Could you check a few things on this model? Use its own coordinates, in mm. A direction names the side the tool comes from. Coordinates: 2 decimals unless noted, no trailing zeros. Order: outer loops, then holes, each group sorted by start corner. A loop starts at its lowest first (then second) coordinate and runs counter-clockwise, first axis right, second up. Notation, with made-up numbers: (88.5, 31) -> (135.5, 31) arc R29 cw to (135.5, 62) -> close; hole circle Ø7 at (-19, 32). An arc over 180 degrees is marked (long way). Use a Markdown table: item, result. Add a question column.
1) If I drill on L1, parallel to Y at x = 0, z = 1.2; L2, parallel to X at y = 0, z = 6.75 (3 decimals), over which ranges is the centre line in solid material (lowest first)? Write a range as [from, to].
2) If we section it at A-A (z = 4): Write out the boundary of the cut face in (x, y) (3 decimals).
3) If we section it at B-B (x = 9.5): Write out the boundary of the cut face in (y, z).
4) Which directions (+Z, -Z, +X, -X, +Y, -Y) give clear straight access to the entire face, cutting with the end or side of a thin tool? Please do faces 4 (the flat face through (30, 0, 15.7)), 5 (the flat face through (8.326, -31.545, 8.381)).
5) Will these pins go through, and if not, where does the flat tip stop? pin 1 Ø1.5 at (x, y) = (-11, 26) entering from -Z; pin 2 Ø2 at (y, z) = (-18, 6.5) entering from +X; pin 3 Ø6 at (x, z) = (24.5, 14.5) entering from -Y; pin 4 Ø5 at (x, z) = (18, 9.5) entering from +Y.
6) If we section it at D-D (y = -27.5): Write out the boundary of the cut face in (x, z), plus the area to 3 significant figures.
7) Thinking about a two-plate mould opening in X: for faces 1 (the flat face through (0, 30, 17)), 2 (the flat face through (8.562, 31.482, 8.381)), 3 (the cylindrical face through (-13.73, -3.52, 0.74)), which applies, +X half, -X half, draft (parallel to the pull), parting line (faces both ways), or undercut?
8) If we section it at C-C (y = -13): Write out the boundary of the cut face in (x, z).
```python
from build123d import *

# Parameters (mm, degrees)
SKETCH_R           = 5.5
SKETCH_R_2         = 4
PAD_DEPTH          = 17
SKETCH001_R        = 31.125
HOLE_DEPTH         = 15.5
PAD001_DEPTH       = 1.3
POLARPATTERN_COUNT = 4


with BuildPart() as part:
    # Sketch → Pad (new body)
    with BuildSketch(Plane.XY):
        Polygon((-29.250775, 16.887943), (-33.775885, 0), (-29.250775, -16.887943), (-16.887943, -29.250775), (0, -33.775885), (16.887943, -29.250775), (29.250775, -16.887943), (33.775885, 0), (29.250775, 16.887943), (16.887943, 29.250775), (0, 33.775885), (-16.887943, 29.250775), align=None)
        with Locations((0, 12.45)):
            Circle(SKETCH_R, mode=Mode.SUBTRACT)
        with Locations((10.782016, -6.225)):
            Circle(SKETCH_R_2, mode=Mode.SUBTRACT)
        with Locations((-10.782016, -6.225)):
            Circle(SKETCH_R_2, mode=Mode.SUBTRACT)
    extrude(amount=PAD_DEPTH)

    # Sketch001 (on Face17 of Pad) → Hole (cut)
    with BuildSketch(Plane.XY.offset(17)):
        Circle(SKETCH001_R)
    extrude(amount=-HOLE_DEPTH, mode=Mode.SUBTRACT)

    # Sketch002 (on Face5 of Hole) → Pad001 (join)
    with BuildSketch(Plane.XY.offset(17)):
        with BuildLine():
            ThreePointArc((-30.866902, 4), (-31.125, 0), (-30.866902, -4))
            Line((-30.866902, -4), (-29.581931, -3.8))
            ThreePointArc((-29.581931, 3.8), (-29.825, 0), (-29.581931, -3.8))
            Line((-30.866902, 4), (-29.581931, 3.8))
        make_face()
    pad001 = extrude(amount=-PAD001_DEPTH)

    # PolarPattern: Pad001 ×4 about axis
    polarpattern_axis = Axis((0, 0, 17), (0, 0, 1))
    for i in range(1, POLARPATTERN_COUNT):
        add(pad001.rotate(polarpattern_axis, i * 360 / POLARPATTERN_COUNT))


solid = part.part
```
Answer sheet:
| question | item | result |
|---|---|---|
| 1 | L1 | [-33.78, 6.95], [17.95, 33.78] |
| 1 | L2 | [-33.776, -31.125], [31.125, 33.776] |
| 2 | outline | (-33.776, 0) -> (-29.251, -16.888) -> (-16.888, -29.251) -> (0, -33.776) -> (16.888, -29.251) -> (29.251, -16.888) -> (33.776, 0) -> (29.251, 16.888) -> (16.888, 29.251) -> (0, 33.776) -> (-16.888, 29.251) -> (-29.251, 16.888) -> close; hole circle Ø62.25 at (0, 0) |
| 3 | outline | (-31.23, 0) -> (-10.01, 0) -> (-10.01, 1.5) -> (-29.64, 1.5) -> (-29.64, 17) -> (-31.23, 17) -> close; (-2.44, 0) -> (31.23, 0) -> (31.23, 17) -> (29.64, 17) -> (29.64, 1.5) -> (-2.44, 1.5) -> close |
| 4 | face 4 | none |
| 4 | face 5 | +Z, -Z, +X, -Y |
| 5 | pin 1 | z = 0 |
| 5 | pin 2 | x = 29.14 |
| 5 | pin 3 | y = -24.64 |
| 5 | pin 4 | y = 29.62 |
| 6 | outline | (-18.64, 0) -> (18.64, 0) -> (18.64, 17) -> (14.58, 17) -> (14.58, 1.5) -> (-14.58, 1.5) -> (-14.58, 17) -> (-18.64, 17) -> close |
| 6 | area | 182 mm2 |
| 7 | face 1 | draft |
| 7 | face 2 | +X half |
| 7 | face 3 | undercut |
| 8 | outline | (-30.29, 0) -> (30.29, 0) -> (30.29, 17) -> (28.28, 17) -> (28.28, 1.5) -> (-28.28, 1.5) -> (-28.28, 17) -> (-30.29, 17) -> close |
